from build123d import *

# Parameters (mm, degrees)
SKETCH1_R                           = 30
BOSS_EXTRUDE1_DEPTH                 = 55
SKETCH3_R                           = 17
HUB_POCKET_DEPTH                    = 7
SKETCH2_W                           = 53.984190988
SKETCH2_H                           = 22
SERVO_POCKET_DEPTH                  = 50
SERVO_FRONT_MOUNT_REACH             = 71.462
SERVO_FRONT_MOUNT_DIRECTION_2_REACH = 71.462
WIRE_ACCESS_DEPTH                   = 11


with BuildPart() as part:
    # Sketch1 → Boss-Extrude1 (new body)
    with BuildSketch(Plane(origin=(0, 0, 0), x_dir=(1, 0, 0), z_dir=(0, 1, 0))):
        with Locations(Location((0, 0, 0), (0, 0, 270))):
            Circle(SKETCH1_R)
    extrude(amount=BOSS_EXTRUDE1_DEPTH)

    # Sketch3 → hub pocket (cut)
    with BuildSketch(Plane(origin=(0, 55, 0), x_dir=(1, 0, 0), z_dir=(0, 1, 0))):
        with Locations(Location((0, 0, 0), (0, 0, 270))):
            Circle(SKETCH3_R)
    extrude(amount=-HUB_POCKET_DEPTH, mode=Mode.SUBTRACT)

    # Sketch2 → servo pocket (cut)
    with BuildSketch(Plane(origin=(0, 55, 0), x_dir=(1, 0, 0), z_dir=(0, 1, 0))):
        with Locations((-8.992095494, 0)):
            Rectangle(SKETCH2_W, SKETCH2_H)
    extrude(amount=-SERVO_POCKET_DEPTH, mode=Mode.SUBTRACT)

    # Servo front mount: up to this face of the body (flat: up to its plane)
    servo_front_mount_end = Plane(part.part.faces().sort_by_distance((-5.380622048, 28.154550276, -11))[0])
    # Sketch4 → Servo front mount (add, up to the picked face)
    with BuildSketch(Plane.XY, mode=Mode.PRIVATE) as servo_front_mount_sk1:
        Polygon((18, 32.5), (11, 32.5), (11, 27.5), (18, 15.375644347), align=None)
    servo_front_mount_tool1 = split(extrude(servo_front_mount_sk1.sketch, amount=-SERVO_FRONT_MOUNT_REACH, mode=Mode.PRIVATE), bisect_by=servo_front_mount_end, keep=Keep.BOTH, mode=Mode.PRIVATE)
    add(servo_front_mount_tool1.solids().sort_by(Axis((15.139344, 26.415223, 0), (0, 0, -1)))[0])

    # Servo front mount direction 2: up to this face of the body (flat: up to its plane)
    servo_front_mount_direction_2_end = Plane(part.part.faces().sort_by_distance((-5.380622048, 28.154550276, 11))[0])
    # Sketch4 → Servo front mount direction 2 (add, up to the picked face)
    with BuildSketch(Plane.XY, mode=Mode.PRIVATE) as servo_front_mount_direction_2_sk1:
        Polygon((18, 32.5), (11, 32.5), (11, 27.5), (18, 15.375644347), align=None)
    servo_front_mount_direction_2_tool1 = split(extrude(servo_front_mount_direction_2_sk1.sketch, amount=SERVO_FRONT_MOUNT_DIRECTION_2_REACH, mode=Mode.PRIVATE), bisect_by=servo_front_mount_direction_2_end, keep=Keep.BOTH, mode=Mode.PRIVATE)
    add(servo_front_mount_direction_2_tool1.solids().sort_by(Axis((15.139344, 26.415223, 0), (0, 0, 1)))[0])

    # Sketch5 → Wire access (cut, symmetric)
    with BuildSketch(Plane.XY):
        Polygon((18, 15.375644347), (23.990381057, 5), (18, 5), align=None)
    extrude(amount=WIRE_ACCESS_DEPTH, both=True, mode=Mode.SUBTRACT)


solid = part.part
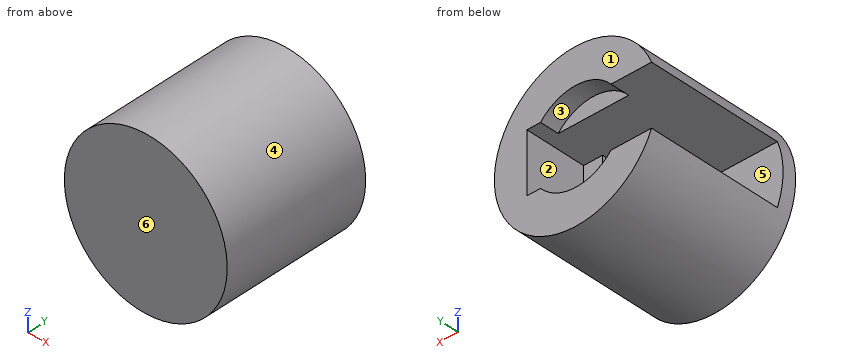
Read the model definition and answer for the solid it produces. Units are mm, in the model's axes. Face numbers are marked on the shaded views. A direction names the side the tool comes from. Coordinates: 2 decimals unless noted, no trailing zeros. Write each loop counter-clockwise with the first axis right and the second up, starting at its lowest first coordinate (ties: lowest second). Pieces come first, ordered by that corner, then holes. Notation, with made-up numbers: (32, -1.75) -> (87, -1.75) arc R13 cw to (87, 13.25) -> close; hole circle Ø8 at (-11.5, -8). An arc over 180 degrees is marked (long way). Return JSON: item names as keys, results as strings.
(1) Each of these flat-tipped pins is pushed along its axis until it touches: P1, Ø3, axis at x = -8, y = 24, coming from the +Z side; P2, Ø6.5, axis at x = -10, z = 4, coming from the +Y side; P3, Ø12, axis at x = 23.5, y = 8.5, coming from the +Z side; P4, Ø5, axis at x = 3.5, z = 15, coming from the +Y side. Where does it stop, or does it pass through?
Answers below:
{"P1": "z = 29.29", "P2": "y = 5", "P3": "z = 24.37", "P4": "y = 55"}
(2) The part is cut by section D-D on z = -12.5. Give the vertices of the cut face in (x, y), then the cut area to 3 significant figures.
Answers below:
{"outline": "(-27.27, 0) -> (27.27, 0) -> (27.27, 55) -> (11.52, 55) -> (11.52, 48) -> (-11.52, 48) -> (-11.52, 55) -> (-27.27, 55) -> close", "area": "2,840 mm^2"}
(3) For a pull along Z with two mould halves and no side action, classify the marked faces 1, 2, 3 and 4 as pulls with the +Z half, pulls with the -Z half, needs draft (parallel to the pull), parting line crosses it, or undercut.
Answers below:
{"face 1": "needs draft", "face 2": "undercut", "face 3": "undercut", "face 4": "parting line crosses it"}
(4) Consider line 1 along Y through (x, z) = (7, 10); line 2 along Z through (x, y) = (10.5, 52.5); line 3 along Z through (x, y) = (-23.5, 30). Determine where each line is inside the solid, lowest interval first. Write a range as from..to.
Answers below:
{"line 1": "0..5", "line 2": "-28.1..-13.37, 13.37..28.1", "line 3": "-18.65..-11, 11..18.65"}
(5) The part is cut by section B-B on z = 0. Give the vertices of the cut face in (x, y), then the cut area to 3 significant figures.
Answers below:
{"outline": "(-30, 0) -> (30, 0) -> (30, 55) -> (18, 55) -> (18, 32.5) -> (11, 32.5) -> (11, 27.5) -> (23.99, 5) -> (-30, 5) -> close", "area": "946 mm^2"}
(6) The part is cut by section C-C on y = 36.5. Give the vertices of the cut face in (x, z).
Answers below:
{"outline": "(-27.91, -11) arc R30 ccw (long way) to (-27.91, 11) -> (18, 11) -> (18, -11) -> close"}
(7) The part is cut by section A-A on x = 0. Give the vertices of the cut face in (y, z).
Answers below:
{"outline": "(0, -30) -> (55, -30) -> (55, -17) -> (48, -17) -> (48, -11) -> (5, -11) -> (5, 11) -> (48, 11) -> (48, 17) -> (55, 17) -> (55, 30) -> (0, 30) -> close"}
(8) Which of the six approach directions +Z, -Z, +X, -X, +Y, -Y give full straight-line access (tool end or side, diameter ignored) to the marked faces 5 and 6?
Answers below:
{"face 5": "-X", "face 6": "+Z, -Z, +X, -X, -Y"}
